For this review, take the finished solid that the model builds, in its own axes (mm). Coordinates: 2 decimals unless noted, no trailing zeros. Order: outer loops, then holes, each group sorted by start corner. A loop starts at its lowest first (then second) coordinate and runs counter-clockwise, first axis right, second up.
from build123d import *

# Parameters (mm, degrees)
F0_W     = 304.8
F0_H     = 152.4
F0_R     = 2.05
F0_R_2   = 4.05
F0_R_3   = 3.05
F1_DEPTH = 3


with BuildPart() as f1:
    # F0 (on Top) → F1 (new body)
    with BuildSketch(Plane.XY):
        Rectangle(F0_W, F0_H)
        with Locations((-139.7, -12.4968)):
            Circle(F0_R, mode=Mode.SUBTRACT)
        with Locations((-139.7, 12.4968)):
            Circle(F0_R, mode=Mode.SUBTRACT)
        with Locations((-50.8, 0)):
            Circle(F0_R_2, mode=Mode.SUBTRACT)
        with Locations((101.6, 0)):
            Circle(F0_R_3, mode=Mode.SUBTRACT)
    extrude(amount=F1_DEPTH)


solid = f1.part
1. Take a section at A-A, the plane x = 101.6. Give the boundary of the cut face in (y, z), plus the area to 3 significant figures.
Answer below:
outline: (-76.2, 0) - (-3.05, 0) - (-3.05, 3) - (-76.2, 3) - close; (3.05, 0) - (76.2, 0) - (76.2, 3) - (3.05, 3) - close
area: 439 mm2
2. The part is to be moulded in two halves that separate along Y. For faces 1 (the face through (-2, 1, 0)), 2 (the face through (-46.94, 1.22, 1.48)), say which applies: +Y half, -Y half, draft (parallel to the pull), parting line (faces both ways), or undercut.
Answer below:
face 1: draft
face 2: undercut
3. Take a section at C-C, the plane x = -50.8. Give the boundary of the cut face in (y, z).
Answer below:
outline: (-76.2, 0) - (-4.05, 0) - (-4.05, 3) - (-76.2, 3) - close; (4.05, 0) - (76.2, 0) - (76.2, 3) - (4.05, 3) - close
4. To check wall thickness, follow L1, parallel to Y at x = -139.7, z = 1.5; L2, parallel to Y at x = -50.8, z = 1.1; L3, parallel to Y at x = 103.5, z = 2.85. State the ranges of each line that lie inside material, in increasing order.
Answer below:
L1: y = -76.2 to -14.55, -10.45 to 10.45, 14.55 to 76.2
L2: y = -76.2 to -4.05, 4.05 to 76.2
L3: y = -76.2 to -2.39, 2.39 to 76.2
5. Take a section at B-B, the plane y = 0. Give the boundary of the cut face in (x, z).
Answer below:
outline: (-152.4, 0) - (-54.85, 0) - (-54.85, 3) - (-152.4, 3) - close; (-46.75, 0) - (98.55, 0) - (98.55, 3) - (-46.75, 3) - close; (104.65, 0) - (152.4, 0) - (152.4, 3) - (104.65, 3) - close
